from build123d import *

# Parameters (mm, degrees)
F1_DEPTH = 6.35


with BuildPart() as f1:
    # F0 (on Top) → F1 (new body)
    with BuildSketch(Plane.XY):
        with BuildLine():
            Line((-20.410651, -17.330817), (-20.410651, 24.579183))
            Line((-20.410651, 24.579183), (4.989349, 24.579183))
            Line((4.989349, 24.579183), (4.989349, -17.330817))
            ThreePointArc((4.989349, -17.330817), (5.733297, -19.126869), (7.529349, -19.870817))
            Line((7.529349, -19.870817), (8.799349, -19.870817))
            ThreePointArc((8.799349, -19.870817), (10.5954, -19.126869), (11.339349, -17.330817))
            Line((11.339349, -17.330817), (11.339349, 28.389183))
            ThreePointArc((11.339349, 28.389183), (10.5954, 30.185234), (8.799349, 30.929183))
            Line((8.799349, 30.929183), (-24.220651, 30.929183))
            ThreePointArc((-24.220651, 30.929183), (-26.016703, 30.185234), (-26.760651, 28.389183))
            Line((-26.760651, 28.389183), (-26.760651, -17.330817))
            ThreePointArc((-26.760651, -17.330817), (-26.016703, -19.126869), (-24.220651, -19.870817))
            Line((-24.220651, -19.870817), (-22.950651, -19.870817))
            ThreePointArc((-22.950651, -19.870817), (-21.1546, -19.126869), (-20.410651, -17.330817))
        make_face()
    extrude(amount=F1_DEPTH)


solid = f1.part
Verification items for the finished model (mm, model axes). A direction names the side the tool comes from. Coordinates: 2 decimals unless noted, no trailing zeros. Order: outer loops, then holes, each group sorted by start corner. A loop starts at its lowest first (then second) coordinate and runs counter-clockwise, first axis right, second up. Notation, with made-up numbers: M 74,-12 L 93,-12 A12 cw 93,-6 Z; hole C 77.5,71 d2. An arc over 180 degrees is marked long. One line per item, written item: value. Start each with the question number.
Item 1: Scan lines: probe 1 along X at (y, z) = (23, 3.5); probe 2 along Y at (x, z) = (-11.5, 5.75). Record each from-to range of solid material in increasing order.
Item 2: Sectioned sample at C-C (x = 2). Enter the section's corners in (y, z).
Item 3: Mould release check, pull along X, two halves, no side actions. Record for faces 1 (the cylindrical face through (-21.174, -19.147, 3.131)), 2 (the flat face through (-21, 12, 6.35)), 3 (the cylindrical face through (10.615, 30.165, 3.131)): released by +X, released by -X, zero draft, split by the parting line, or undercut.
Item 4: Gauge pin test, flat end, axial feed: pin 1 (1 mm diameter, centred on x = -17.5, z = 5.5, fed in from -Y). Record the tip position at first contact, or that the pin passes through.
Item 5: Sectioned sample at B-B (z = 5.5). Enter the section's corners in (x, y).
Item 6: Sectioned sample at A-A (y = 23). Enter the section's corners in (x, z), then the cut area to 3 significant figures.
Item 7: Access from +Z, -Z, +X, -X, +Y, -Y to the whole of each face (thin tool, end or side, straight path). Record for faces 4 (the flat face through (-7, 30.929, 3)), 5 (the flat face through (-8, 24.579, 3)).
Conclusion:
1. probe 1: x = -26.76 to -20.41, 4.99 to 11.34
1. probe 2: y = 24.58 to 30.93
2. outline: M 24.58,0 L 30.93,0 L 30.93,6.35 L 24.58,6.35 Z
3. face 1: undercut
3. face 2: zero draft
3. face 3: released by +X
4. pin 1: stops at y = 24.58
5. outline: M -26.76,-17.33 A2.54 ccw -24.22,-19.87 L -22.95,-19.87 A2.54 ccw -20.41,-17.33 L -20.41,24.58 L 4.99,24.58 L 4.99,-17.33 A2.54 ccw 7.53,-19.87 L 8.8,-19.87 A2.54 ccw 11.34,-17.33 L 11.34,28.39 A2.54 ccw 8.8,30.93 L -24.22,30.93 A2.54 ccw -26.76,28.39 Z
6. outline: M -26.76,0 L -20.41,0 L -20.41,6.35 L -26.76,6.35 Z; M 4.99,0 L 11.34,0 L 11.34,6.35 L 4.99,6.35 Z
6. area: 80.6 mm^2
7. face 4: +Z, -Z, +X, -X, +Y
7. face 5: +Z, -Z, -Y
